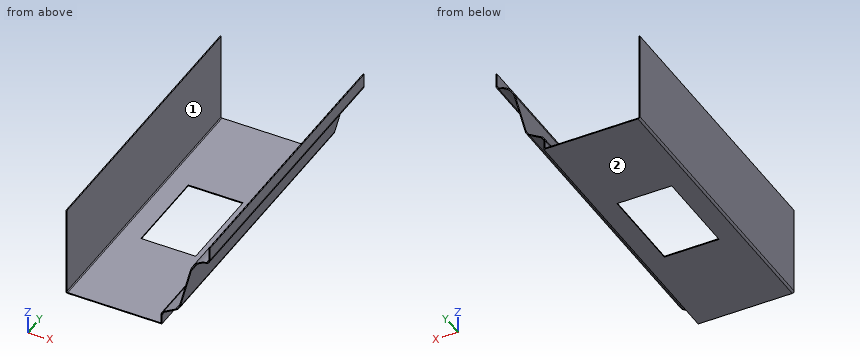
```python
from build123d import *

# Parameters (mm, degrees)
F1_DEPTH = 300
F2_W     = 57
F2_H     = 92
F3_DEPTH = 25
F4_DEPTH = 25
F5_DEPTH = 25


with BuildPart() as f1:
    # F0 (on Front) → F1 (new body)
    with BuildSketch(Plane.XZ):
        with BuildLine():
            Line((75, 38.914216), (75, 52.5))
            Line((75, 52.5), (74, 52.5))
            Line((74, 52.5), (74, 38.875))
            ThreePointArc((74, 38.875), (73.361451, 36.706903), (71.649678, 35.231024))
            ThreePointArc((71.649678, 35.231024), (60.8185, 29.988223), (54.643786, 19.659898))
            Line((54.643786, 19.659898), (43.416317, -24.63337))
            ThreePointArc((43.416317, -24.63337), (41.948954, -27.705545), (39.413109, -29.977308))
            Line((39.413109, -29.977308), (26.950339, -37.332837))
            ThreePointArc((26.950339, -37.332837), (24.789532, -39.524934), (24, -42.5))
            Line((24, -42.5), (24, -51.5))
            Line((24, -51.5), (-73, -51.5))
            ThreePointArc((-73, -51.5), (-73.707107, -51.207107), (-74, -50.5))
            Line((-74, -50.5), (-74, 42.5))
            Line((-74, 42.5), (-75, 42.5))
            Line((-75, 42.5), (-75, -50.5))
            ThreePointArc((-75, -50.5), (-74.414214, -51.914214), (-73, -52.5))
            Line((-73, -52.5), (25, -52.5))
            Line((25, -52.5), (25, -42.5))
            ThreePointArc((25, -42.5), (25.657943, -40.020778), (27.458616, -38.194031))
            Line((27.458616, -38.194031), (39.921386, -30.838502))
            ThreePointArc((39.921386, -30.838502), (42.749295, -28.305091), (44.385661, -24.87908))
            Line((44.385661, -24.87908), (55.613129, 19.414189))
            ThreePointArc((55.613129, 19.414189), (61.539869, 29.29273), (71.932405, 34.263346))
            ThreePointArc((71.932405, 34.263346), (74.173992, 36.121942), (75, 38.914216))
        make_face()
    extrude(amount=F1_DEPTH)

    # F2 (on face) → F3 (cut)
    with BuildSketch(Plane(origin=(0, 0, -52.5), x_dir=(1, 0, 0), z_dir=(0, 0, -1))):
        with Locations((-24, 150)):
            Rectangle(F2_W, F2_H)
    extrude(amount=-F3_DEPTH, mode=Mode.SUBTRACT)

    # F2 (on face) → F4 (cut)
    with BuildSketch(Plane(origin=(0, 0, -52.5), x_dir=(1, 0, 0), z_dir=(0, 0, -1))):
        with Locations((-24, 150)):
            Rectangle(F2_W, F2_H)
    extrude(amount=-F4_DEPTH, mode=Mode.SUBTRACT)

    # F2 (on face) → F5 (cut)
    with BuildSketch(Plane(origin=(0, 0, -52.5), x_dir=(1, 0, 0), z_dir=(0, 0, -1))):
        with Locations((-24, 150)):
            Rectangle(F2_W, F2_H)
    extrude(amount=-F5_DEPTH, mode=Mode.SUBTRACT)


solid = f1.part
```
Could you check a few things on this model? Use its own coordinates, in mm. Face numbers are marked on the shaded views. A direction names the side the tool comes from. Round coordinates to 2 decimals unless told otherwise and drop trailing zeros. Write each loop counter-clockwise with the first axis right and the second up, starting at its lowest first coordinate (ties: lowest second). Pieces come first, ordered by that corner, then holes.
(1) For pin 1 (1.1 mm diameter, centred on x = -74.5, y = -81, fed in from +Z); pin 2 (0.8 mm diameter, centred on y = -152.5, z = -52, fed in from +X); pin 3 (1 mm diameter, centred on x = 13, y = -91.5, fed in from +Z), each with a flat end and sliding along its axis, tell me the tip position at first contact or that it passes through.
Findings below:
pin 1: stops at z = 42.5
pin 2: stops at x = 25
pin 3: stops at z = -51.5
(2) Suppose I cut it at D-D on z = -2. Write out the boundary of the cut face in (x, y).
Findings below:
outline: (-75, -300) - (-74, -300) - (-74, 0) - (-75, 0) - close; (49.15, -300) - (50.19, -300) - (50.19, 0) - (49.15, 0) - close
(3) Suppose I cut it at B-B on x = -6.5. Write out the boundary of the cut face in (y, z), and give its area (3 significant figures).
Findings below:
outline: (-300, -52.5) - (-196, -52.5) - (-196, -51.5) - (-300, -51.5) - close; (-104, -52.5) - (0, -52.5) - (0, -51.5) - (-104, -51.5) - close
area: 208 mm2
(4) Suppose I cut it at A-A on y = -129. Write out the boundary of the cut face in (x, z) (1 decimal).
Findings below:
outline: (-75, -50.5) arc R2 ccw to (-73, -52.5) - (-52.5, -52.5) - (-52.5, -51.5) - (-73, -51.5) arc R1 cw to (-74, -50.5) - (-74, 42.5) - (-75, 42.5) - close; (4.5, -52.5) - (25, -52.5) - (25, -42.5) arc R5 cw to (27.5, -38.2) - (39.9, -30.8) arc R9.7 ccw to (44.4, -24.9) - (55.6, 19.4) arc R20 cw to (71.9, 34.3) arc R5 ccw to (75, 38.9) - (75, 52.5) - (74, 52.5) - (74, 38.9) arc R4 cw to (71.6, 35.2) arc R21 ccw to (54.6, 19.7) - (43.4, -24.6) arc R8.7 cw to (39.4, -30) - (27, -37.3) arc R6 ccw to (24, -42.5) - (24, -51.5) - (4.5, -51.5) - close
(5) If I drill on probe 1 along X at (y, z) = (-285.5, -43.5); probe 2 along Z at (x, y) = (-63.5, -273); probe 3 along X at (y, z) = (-118.5, 47.5), over which ranges is the centre line in solid material (lowest first)?
Findings below:
probe 1: x = -75 to -74, 24 to 25
probe 2: z = -52.5 to -51.5
probe 3: x = 74 to 75
(6) Which directions (+Z, -Z, +X, -X, +Y, -Y) give clear straight access to the entire face, cutting with the end or side of a thin tool? Please do the marked faces 1 and 2.
Findings below:
face 1: +Z, +Y, -Y
face 2: -Z, +X, -X, +Y, -Y
(7) Suppose I cut it at C-C on y = -97.5. Write out the boundary of the cut face in (x, z) (1 decimal), and give its area (3 significant figures).
Findings below:
outline: (-75, -50.5) arc R2 ccw to (-73, -52.5) - (25, -52.5) - (25, -42.5) arc R5 cw to (27.5, -38.2) - (39.9, -30.8) arc R9.7 ccw to (44.4, -24.9) - (55.6, 19.4) arc R20 cw to (71.9, 34.3) arc R5 ccw to (75, 38.9) - (75, 52.5) - (74, 52.5) - (74, 38.9) arc R4 cw to (71.6, 35.2) arc R21 ccw to (54.6, 19.7) - (43.4, -24.6) arc R8.7 cw to (39.4, -30) - (27, -37.3) arc R6 ccw to (24, -42.5) - (24, -51.5) - (-73, -51.5) arc R1 cw to (-74, -50.5) - (-74, 42.5) - (-75, 42.5) - close
area: 318 mm2
